from build123d import *

# Parameters (mm, degrees)
SKETCH1_W                = 7.2
SKETCH1_H                = 5.6
BODY_DEPTH               = 6.4
BODY_CHAMFER_SIZE        = 0.1
SKETCH2_R                = 1.725
MOUNT_DEPTH              = 4
SKETCH3_W                = 1.45
SKETCH3_H                = 5
MOUNT_RAILS_DEPTH        = 3
SKETCH4_R                = 2.25
BODY_CUT_1_DEPTH         = 4.8
SKETCH5_W                = 5.6
SKETCH5_H                = 5.6
BODY_CUT_2_DEPTH         = 2.5
SKETCH6_R                = 0.975
POLE_DEPTH               = 7.3
POLE_CHAMFER_SIZE        = 0.5
POLE_CHAMFER_SIZE2       = 0.2
SKETCH7_W                = 1.99
SKETCH7_H                = 5
RIGHT_RAIL_DEPTH         = 0.7
RIGHT_RAIL_CHAMFER_SIZE  = 0.4
RIGHT_RAIL_CHAMFER_SIZE2 = 1
LEFT_RAIL_CHAMFER_SIZE   = 1
LEFT_RAIL_CHAMFER_SIZE2  = 0.4
RIGHT_LEG_DEPTH          = 0.75


with BuildPart() as part:
    # Sketch1 → Body (new body)
    with BuildSketch(Plane(origin=(0, 0, 0), x_dir=(1, 0, 0), z_dir=(0, 1, 0))):
        Rectangle(SKETCH1_W, SKETCH1_H)
    extrude(amount=BODY_DEPTH)

    # Body Chamfer
    body_chamfer_edges = [part.edges().sort_by_distance(p)[0] for p in [
        (-3.6, 6.4, 0),
        (0, 6.4, 2.8),
        (3.6, 6.4, 0),
        (0, 6.4, -2.8),
    ]]
    chamfer(body_chamfer_edges, length=BODY_CHAMFER_SIZE)

    # Sketch2 → Mount (add)
    with BuildSketch(Plane(origin=(0, 6.4, 0), x_dir=(1, 0, 0), z_dir=(0, 1, 0))):
        Circle(SKETCH2_R)
    extrude(amount=MOUNT_DEPTH)

    # Sketch3 → Mount Rails (add)
    with BuildSketch(Plane(origin=(0, 6.4, 0), x_dir=(1, 0, 0), z_dir=(0, 1, 0))):
        Rectangle(SKETCH3_W, SKETCH3_H)
    extrude(amount=MOUNT_RAILS_DEPTH)

    # Sketch4 → Body Cut 1 (cut)
    with BuildSketch(Plane.XZ):
        Circle(SKETCH4_R)
    extrude(amount=-BODY_CUT_1_DEPTH, mode=Mode.SUBTRACT)

    # Sketch5 → Body Cut 2 (cut)
    with BuildSketch(Plane.XZ):
        Rectangle(SKETCH5_W, SKETCH5_H)
    extrude(amount=-BODY_CUT_2_DEPTH, mode=Mode.SUBTRACT)

    # Sketch6 → Pole (add)
    with BuildSketch(Plane.XZ.offset(-4.8)):
        Circle(SKETCH6_R)
    extrude(amount=POLE_DEPTH)

    # Pole Chamfer
    pole_chamfer_edges = [part.edges().sort_by_distance(p)[0] for p in [
        (-0.975, -2.5, 0),
    ]]
    pole_chamfer_side = [part.faces().sort_by_distance(p)[0] for p in [
        (-0.975, 1.15, 0),
    ]]
    chamfer(pole_chamfer_edges, length=POLE_CHAMFER_SIZE, length2=POLE_CHAMFER_SIZE2, reference=pole_chamfer_side[0])

    # Sketch7 → Right Rail (add)
    with BuildSketch(Plane(origin=(3.6, 0, 0), x_dir=(0, 0, -1), z_dir=(1, 0, 0))):
        with Locations((0, 2.5)):
            Rectangle(SKETCH7_W, SKETCH7_H)
    right_rail = extrude(amount=RIGHT_RAIL_DEPTH)

    # Rail Mirror: Right Rail across plane
    add(right_rail.mirror(Plane(origin=(0, 0, 0), x_dir=(0, 0, 1), z_dir=(1, 0, 0))))

    # Right Rail Chamfer
    right_rail_chamfer_edges = [part.edges().sort_by_distance(p)[0] for p in [
        (4.3, 0, 0),
    ]]
    right_rail_chamfer_side = [part.faces().sort_by_distance(p)[0] for p in [
        (3.377890346, 0, 0),
    ]]
    chamfer(right_rail_chamfer_edges, length=RIGHT_RAIL_CHAMFER_SIZE, length2=RIGHT_RAIL_CHAMFER_SIZE2, reference=right_rail_chamfer_side[0])

    # Left Rail Chamfer
    left_rail_chamfer_edges = [part.edges().sort_by_distance(p)[0] for p in [
        (-4.3, 0, 0),
    ]]
    left_rail_chamfer_side = [part.faces().sort_by_distance(p)[0] for p in [
        (-4.3, 2.5, 0),
    ]]
    chamfer(left_rail_chamfer_edges, length=LEFT_RAIL_CHAMFER_SIZE, length2=LEFT_RAIL_CHAMFER_SIZE2, reference=left_rail_chamfer_side[0])

    # Sketch8 → Right Leg (add)
    with BuildSketch(Plane(origin=(3.6, 0, 0), x_dir=(0, 0, -1), z_dir=(1, 0, 0))):
        with BuildLine():
            Line((-3.016216216, 2.849166829), (-4.4, -0.036165464))
            ThreePointArc((-4.4, -0.036165464), (-4.221723875, -0.497920402), (-3.759968937, -0.319644277))
            Line((-3.759968937, -0.319644277), (-3.197806774, 0.852521967))
            ThreePointArc((-3.197806774, 0.852521967), (-3.029447088, 1.008649464), (-2.8, 1))
            Line((-2.8, 1), (-2.8, 2.849166829))
            Line((-2.8, 2.849166829), (-3.016216216, 2.849166829))
        make_face()
    right_leg = extrude(amount=-RIGHT_LEG_DEPTH)

    # Leg Mirror: Right Leg across plane
    add(right_leg.mirror(Plane(origin=(0, 0, 0), x_dir=(0, 0, 1), z_dir=(1, 0, 0))))


solid = part.part
Can you work these out from the model? Positions are in its coordinate system, mm. A direction names the side the tool comes from. Give positions to 0.01 mm unless a question says otherwise; leave off trailing zeros. Loops run counter-clockwise (first coordinate to the right, second up) from the corner with the lowest first, then second, coordinate; pieces in that order, holes last. Notation, with made-up numbers: (-10, 46) -> (15, 46) arc R36 cw to (15, 85) -> close; hole circle Ø1 at (-33, 80.25). An arc over 180 degrees is marked (long way). Return JSON: item names as keys, results as strings.
Q1. I want a section at C-C, the plane y = 9. List the corners of the cut face in (x, z) for me (3 decimals).
Checks:
{"outline": "(-0.725, -2.5) -> (0.725, -2.5) -> (0.725, -1.565) arc R1.725 ccw to (0.725, 1.565) -> (0.725, 2.5) -> (-0.725, 2.5) -> (-0.725, 1.565) arc R1.725 ccw to (-0.725, -1.565) -> close"}
Q2. I need wall thicknesses on probe 1 along Z at (x, y) = (0, 3.3) (3 decimals); probe 2 along X at (y, z) = (0.25, 2.75); probe 3 along X at (y, z) = (3.75, 0.75). Which ranges of each line are inside material? Lowest first, please.
Checks:
{"probe 1": "z = -2.8 to -2.25, -0.975 to 0.975, 2.25 to 2.8", "probe 2": "x = -3.6 to -2.8, 2.8 to 3.6", "probe 3": "x = -4.3 to -2.12, -0.62 to 0.62, 2.12 to 4.3"}
Q3. I want a section at B-B, the plane x = 0. List the corners of the cut face in (y, z) for me (3 decimals).
Checks:
{"outline": "(-2.5, -0.775) -> (-2, -0.975) -> (4.8, -0.975) -> (4.8, -2.25) -> (2.5, -2.25) -> (2.5, -2.8) -> (6.3, -2.8) -> (6.4, -2.7) -> (6.4, -2.5) -> (9.4, -2.5) -> (9.4, -1.725) -> (10.4, -1.725) -> (10.4, 1.725) -> (9.4, 1.725) -> (9.4, 2.5) -> (6.4, 2.5) -> (6.4, 2.7) -> (6.3, 2.8) -> (2.5, 2.8) -> (2.5, 2.25) -> (4.8, 2.25) -> (4.8, 0.975) -> (-2, 0.975) -> (-2.5, 0.775) -> close"}
Q4. For pin 1 Ø0.5 at (y, z) = (7.5, 2) entering from +X (3 decimals); pin 2 Ø0.7 at (y, z) = (8, 2) entering from -X (3 decimals); pin 3 Ø0.7 at (x, y) = (0, 7.5) entering from -Z, each with a flat end and sliding along its axis, tell me the tip position at first contact or that it passes through.
Checks:
{"pin 1": "stops at x = 0.725", "pin 2": "stops at x = -0.725", "pin 3": "stops at z = -2.5"}
Q5. We'd pull the mould along X, two halves only. Please class faces 4 (the face through (-0.725, 8, -2)), 5 (the face through (-2.8, 1, 0)), 6 (the face through (-2.85, 1.2, 3.4)), 7 (the face through (4.3, 3, 0)): released by +X, released by -X, zero draft, split by the parting line, or undercut.
Checks:
{"face 4": "released by -X", "face 5": "undercut", "face 6": "undercut", "face 7": "released by +X"}
Q6. I want a section at A-A, the plane y = 3.5. List the corners of the cut face in (x, z) for me (3 decimals).
Checks:
{"outline": "(-4.3, -0.995) -> (-3.6, -0.995) -> (-3.6, -2.8) -> (3.6, -2.8) -> (3.6, -0.995) -> (4.3, -0.995) -> (4.3, 0.995) -> (3.6, 0.995) -> (3.6, 2.8) -> (-3.6, 2.8) -> (-3.6, 0.995) -> (-4.3, 0.995) -> close; circle Ø1.95 at (0, 0); hole circle Ø4.5 at (0, 0)"}
Q7. On a 3-axis mill with a long thin cutter (end or side, diameter ignored), from which of +Z, -Z, +X, -X, +Y, -Y can I reach the whole of each face in a straight line? I mean faces 1 (the face through (1.645, 8.372, -0.518)), 2 (the face through (3, 0, 0)), 3 (the face through (-0.725, 8, 2)). Say none if no direction works.
Checks:
{"face 1": "+Y", "face 2": "-Z, +X, -Y", "face 3": "+Z, -X, +Y"}
